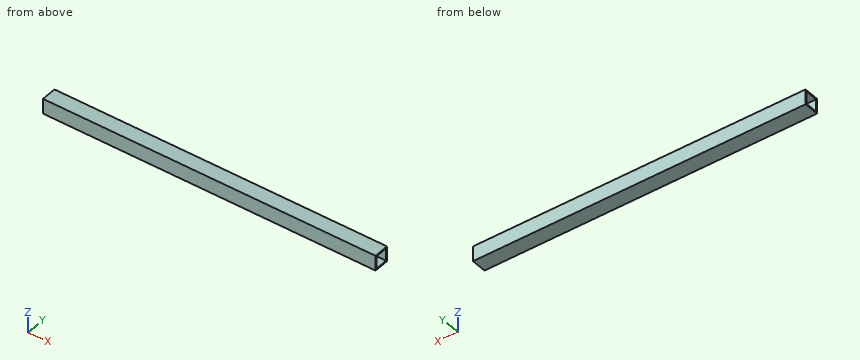
from build123d import *

# Parameters (mm, degrees)
SKETCH1_W               = 838.1
SKETCH1_H               = 38.1
BOSS_EXTRUDE1_DEPTH     = 38.1
SKETCH2_W               = 31.75
SKETCH2_H               = 31.75
CUT_EXTRUDE1_DEPTH      = 1
CUT_EXTRUDE1_DEPTH_BACK = 839.1


with BuildPart() as part:
    # Sketch1 → Boss-Extrude1 (new body)
    with BuildSketch(Plane.XY):
        with Locations((419.05, 19.05)):
            Rectangle(SKETCH1_W, SKETCH1_H)
    extrude(amount=-BOSS_EXTRUDE1_DEPTH)

    # Sketch2 → Cut-Extrude1 (cut, two sides)
    with BuildSketch(Plane(origin=(838.1, 0, 0), x_dir=(0, 0, -1), z_dir=(1, 0, 0))) as cut_extrude1_sk:
        with Locations((19.05, 19.05)):
            Rectangle(SKETCH2_W, SKETCH2_H)
    extrude(amount=CUT_EXTRUDE1_DEPTH, mode=Mode.SUBTRACT)
    extrude(cut_extrude1_sk.sketch, amount=-CUT_EXTRUDE1_DEPTH_BACK, mode=Mode.SUBTRACT)


solid = part.part
Build history of the part. All positions in model axes, mm. Give positions to 0.01 mm unless a question says otherwise; leave off trailing zeros. Loops run counter-clockwise (first coordinate to the right, second up) from the corner with the lowest first, then second, coordinate; pieces in that order, holes last. Notation, with made-up numbers: (80, -6.75) - (95, -6.75) arc R10 ccw to (95, 4.25) - close; hole circle Ø2 at (-17.75, 52.5). An arc over 180 degrees is marked (long way). Write item = value, one per line. Start each with the question number.
1) Band-saw the part on C-C on x = 289.5. Give the cut face in (y, z) (3 decimals).
2) Band-saw the part on B-B on z = -19. Give the cut face in (x, y) (3 decimals), plus the area to 3 significant figures.
3) Drop a flat-ended pin along its axis: pin 1 Ø12 at (y, z) = (23, -10) entering from -X. Give the stop position or say it passes through.
4) Probe probe 1 along Z at (x, y) = (654, 14) (3 decimals); probe 2 along Y at (x, z) = (799, -30.5) (3 decimals). List the from-to ranges inside material, lowest first. Write a range as from..to.
5) Band-saw the part on A-A on y = 28. Give the cut face in (x, z) (3 decimals), plus the area to 3 significant figures.
Final values:
q1.outline = (0, -38.1) - (38.1, -38.1) - (38.1, 0) - (0, 0) - close; hole (3.175, -34.925) - (34.925, -34.925) - (34.925, -3.175) - (3.175, -3.175) - close
q2.outline = (0, 0) - (838.1, 0) - (838.1, 3.175) - (0, 3.175) - close; (0, 34.925) - (838.1, 34.925) - (838.1, 38.1) - (0, 38.1) - close
q2.area = 5,320 mm²
q3.pin_1 = through
q4.probe_1 = -38.1..-34.925, -3.175..0
q4.probe_2 = 0..3.175, 34.925..38.1
q5.outline = (0, -38.1) - (838.1, -38.1) - (838.1, -34.925) - (0, -34.925) - close; (0, -3.175) - (838.1, -3.175) - (838.1, 0) - (0, 0) - close
q5.area = 5,320 mm²
